from build123d import *

# Parameters (mm, degrees)
EXTRUDE1_DEPTH = 75
EXTRUDE2_DEPTH = 108.475952642
EXTRUDE3_DEPTH = 108.475952642


with BuildPart() as part:
    # Sketch1 → Extrude1 (new body)
    with BuildSketch(Plane(origin=(0, 0, 0), x_dir=(1, 0, 0), z_dir=(0, 1, 0))):
        Polygon((-92.5, -15), (-55, -79.951905284), (-119.951905284, -117.451905284), (-157.451905284, -52.5), align=None)
    extrude(amount=EXTRUDE1_DEPTH)

    # Sketch2 → Extrude2 (cut, through all)
    with BuildSketch(Plane(origin=(20.870190528, 0, 36.148230359), x_dir=(0.866025404, 0, -0.5), z_dir=(0.5, 0, 0.866025404))):
        Polygon((-162.60734985, 25), (-125.10734985, 75), (-162.60734985, 75), align=None)
        Polygon((-87.60734985, 75), (-125.10734985, 75), (-87.60734985, 25), align=None)
    extrude(amount=-EXTRUDE2_DEPTH, mode=Mode.SUBTRACT)

    # Sketch3 → Extrude3 (cut, through all)
    with BuildSketch(Plane(origin=(-140.822095812, 0, 81.303674925), x_dir=(0.5, 0, 0.866025404), z_dir=(-0.866025404, 0, 0.5))):
        Polygon((-33.259618943, 75), (4.240381057, 75), (-33.259618943, 25), align=None)
        Polygon((41.740381057, 75), (41.740381057, 25), (4.240381057, 75), align=None)
    extrude(amount=-EXTRUDE3_DEPTH, mode=Mode.SUBTRACT)


solid = part.part
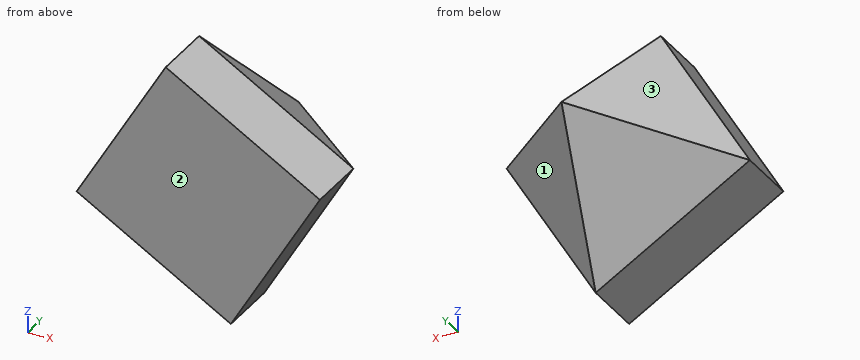
Read the model definition and answer for the solid it produces. Units are mm, in the model's axes. Face numbers are marked on the shaded views. Coordinates: 2 decimals unless noted, no trailing zeros. Write each loop counter-clockwise with the first axis right and the second up, starting at its lowest first coordinate (ties: lowest second). Pieces come first, ordered by that corner, then holes. Notation, with made-up numbers: M 22.25,-20 L 49.25,-20 A13 cw 49.25,3 Z; hole C -28.5,54.5 d1. An arc over 180 degrees is marked long. Use a Markdown table: item, result.
Q1. Straight lines are drawn through the part: L1, parallel to Y at x = -98.5, z = 101; L2, parallel to Z at x = -90, y = 40; L3, parallel to X at y = 11, z = 101. For each, find the intervals that lie inside material, in ascending order. Write a range as [from, to].
Answer block:
| item | result |
|---|---|
| L1 | y = [0, 29.7] |
| L2 | z = [41.83, 87.17] |
| L3 | x = [-129.45, -91.46] |
Q2. The part is cut by section A-A, the plane x = -85.5. Write down the section's boundary in (y, z).
Answer block:
| item | result |
|---|---|
| outline | M 0,27.12 L 25,27.12 L 54.77,71.78 L 25,97.56 L 0,97.56 Z |
Q3. Determine the mould class of the marked faces 1, 2 and 3 for opening direction X: released by +X, released by -X, zero draft, split by the parting line, or undercut.
Answer block:
| item | result |
|---|---|
| face 1 | released by +X |
| face 2 | zero draft |
| face 3 | released by -X |
Q4. The part is cut by section C-C, the plane y = 12. Write down the section's boundary in (x, z).
Answer block:
| item | result |
|---|---|
| outline | M -157.45,52.5 L -92.5,15 L -55,79.95 L -119.95,117.45 Z |
Q5. Each of these flat-tipped pins is pushed along its axis until it touches: pin 1 Ø1.5 at (y, z) = (57.5, 58.5) entering from +X; pin 2 Ø8 at (x, y) = (-80, 39.5) entering from -Z; pin 3 Ø12 at (y, z) = (53.5, 50) entering from -X. Where does it stop, or does it pass through?
Answer block:
| item | result |
|---|---|
| pin 1 | stops at x = -94.75 |
| pin 2 | stops at z = 49.24 |
| pin 3 | stops at x = -124.12 |
Q6. The part is cut by section B-B, the plane z = 62. Write down the section's boundary in (x, y), then the cut area to 3 significant figures.
Answer block:
| item | result |
|---|---|
| outline | M -151.97,0 L -65.36,0 L -65.36,25 L -105.09,70.88 L -122,59.61 L -151.97,25 Z |
| area | 4,280 mm2 |
Q7. The part is cut by section D-D, the plane z = 98.5. Write down the section's boundary in (x, y), then the cut area to 3 significant figures.
Answer block:
| item | result |
|---|---|
| outline | M -130.89,0 L -87.13,0 L -87.13,25 L -114.87,43.5 L -130.89,25 Z |
| area | 1,500 mm2 |
